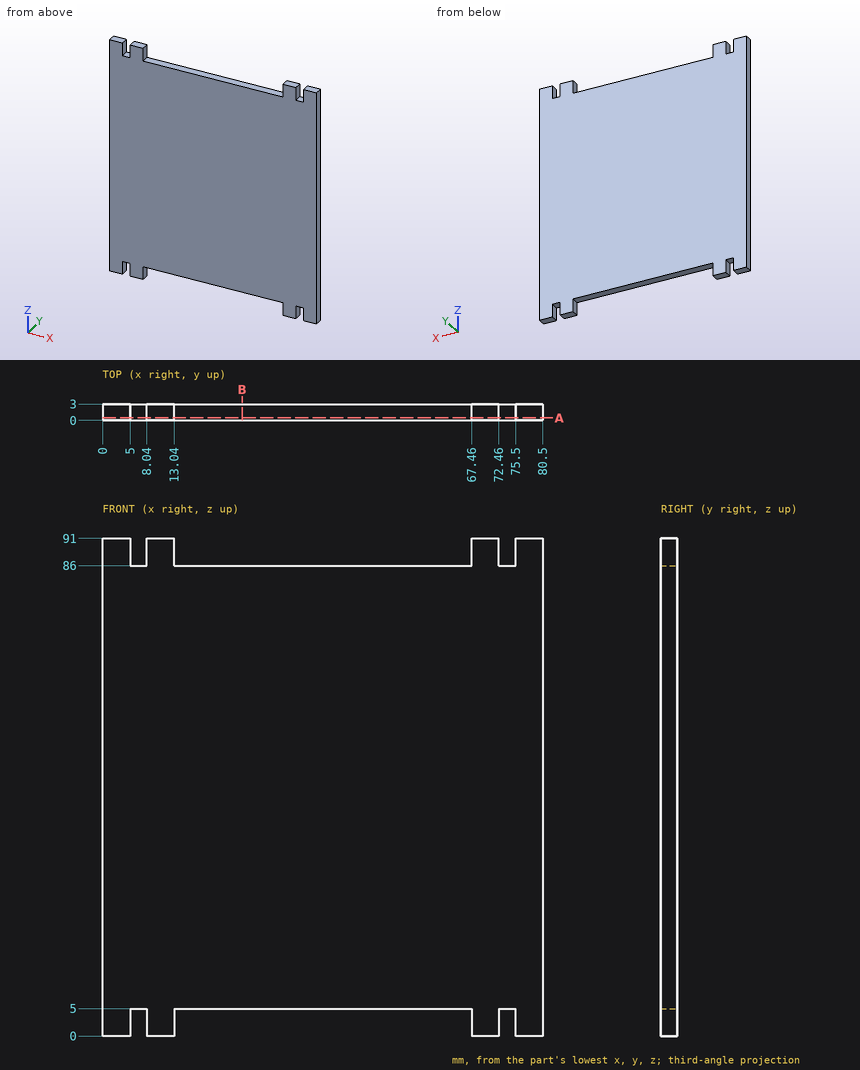
Could you check a few things on this drawing? It's one solid part, dimensions in mm from its lowest x, y, z. Give positions to 0.01 mm unless a question says otherwise; leave off trailing zeros. Write each loop counter-clockwise with the first axis right and the second up, starting at its lowest first coordinate (ties: lowest second). Pieces come first, ordered by that corner, then holes. Notation, with made-up numbers: (23.25, 5) -> (41.25, 5) arc R22 cw to (41.25, 36) -> close; hole circle Ø1 at (-24.75, 30). An arc over 180 degrees is marked (long way). Write item = value, one per line.
(1) Suppose I cut it at A-A on y = 0.45. Write out the boundary of the cut face in (x, z).
Worked out:
outline = (0, 0) -> (5, 0) -> (5, 5) -> (8.04, 5) -> (8.04, 0) -> (13.04, 0) -> (13.04, 5) -> (67.46, 5) -> (67.46, 0) -> (72.46, 0) -> (72.46, 5) -> (75.5, 5) -> (75.5, 0) -> (80.5, 0) -> (80.5, 91) -> (75.5, 91) -> (75.5, 86) -> (72.46, 86) -> (72.46, 91) -> (67.46, 91) -> (67.46, 86) -> (13.04, 86) -> (13.04, 91) -> (8.04, 91) -> (8.04, 86) -> (5, 86) -> (5, 91) -> (0, 91) -> close
(2) I'm going to push flat-ended pins straight in: P1, Ø1.5, axis at x = 6, y = 1.5, coming from the +Z side; P2, Ø1, axis at x = 26, y = 0.5, coming from the -Z side. Where does each tip first touch, or does it pass through?
Worked out:
P1 = 86
P2 = 5
(3) Suppose I cut it at B-B on x = 25.5. Write out the boundary of the cut face in (y, z), then the cut area to 3 significant figures.
Worked out:
outline = (0, 5) -> (3, 5) -> (3, 86) -> (0, 86) -> close
area = 243 mm^2
(4) I need wall thicknesses on probe 1 along Z at (x, y) = (19.5, 1.25). Which ranges of the line are inside material? Lowest first, please. Write a range as from..to.
Worked out:
probe_1 = 5..86
